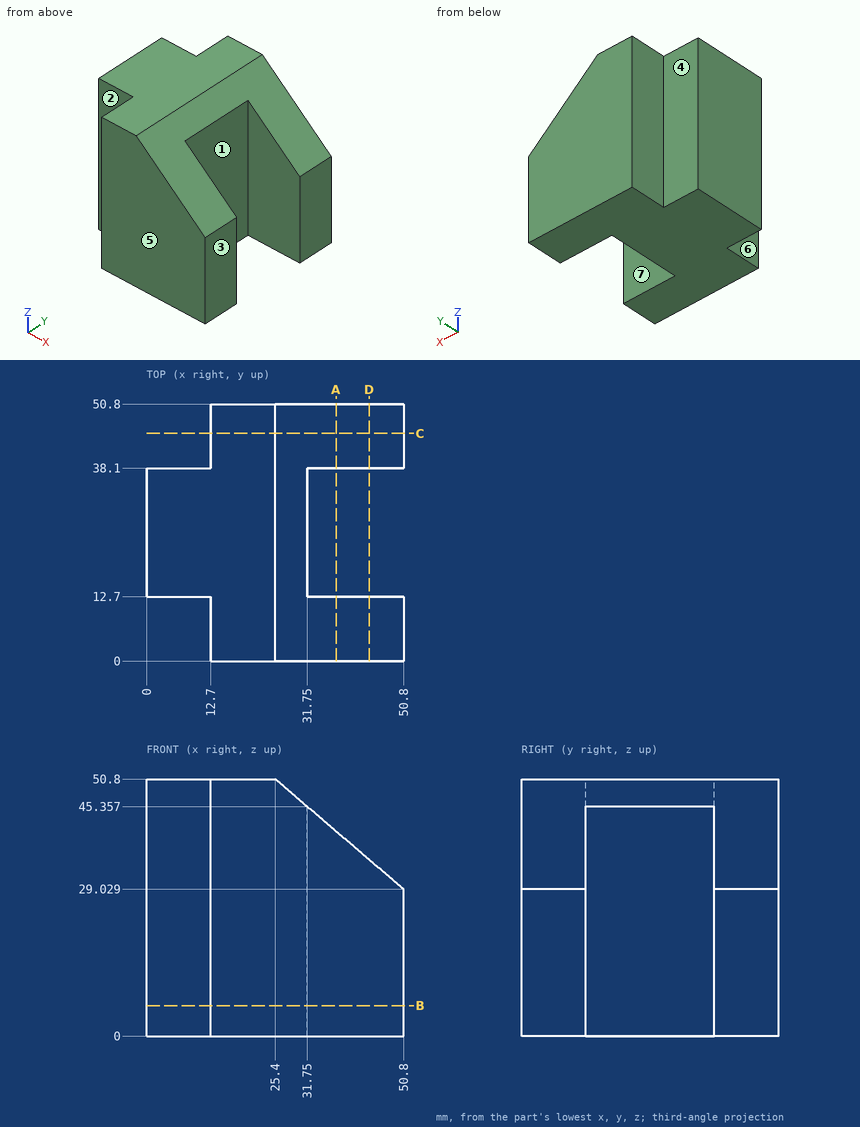
The drawing under review shows one solid part. Ordinate dimensions are in mm from its lowest x, y, z. A direction names the side the tool comes from. Coordinates: 2 decimals unless noted, no trailing zeros. Write each loop counter-clockwise with the first axis right and the second up, starting at its lowest first coordinate (ties: lowest second). Pieces come first, ordered by that corner, then holes. Notation, with made-up numbers: (57, 65) -> (102, 65) arc R28 cw to (102, 89) -> close; hole circle Ø4 at (38.5, -15). An arc over 180 degrees is marked (long way). One line per item, written item: value. Start each with the question number.
Q1. The part is to be moulded in two halves that separate along Y. For the marked faces 1, 2 and 3, say which applies: +Y half, -Y half, draft (parallel to the pull), parting line (faces both ways), or undercut.
Q2. Add section C-C, the plane y = 45. Give the boundary of the cut face in (x, z).
Q3. Clearance check with flat-ended pins moving along their axes: P1, Ø1.5, axis at x = 5.5, z = 25, coming from the +Y side; P2, Ø5, axis at y = 5, z = 27, coming from the -X side; P3, Ø20.5, axis at y = 23, z = 18, coming from the +X side. State where each tip first meets the part, or that it passes through.
Q4. To check wall thickness, follow probe 1 along Y at (x, z) = (44, 19.5); probe 2 along X at (y, z) = (13, 28); probe 3 along X at (y, z) = (7, 4). State the ranges of each line that lie inside material, in increasing order.
Q5. Add section D-D, the plane x = 44. Give the boundary of the cut face in (y, z).
Q6. Add section B-B, the plane z = 6. Give the boundary of the cut face in (x, y), then the cut area to 3 significant figures.
Q7. Add section A-A, the plane x = 37.5. Give the boundary of the cut face in (y, z), then the cut area to 3 significant figures.
Q8. For the marked faces 4, 5, 6 and 7, list the 3-axis set-ups (+Z, -Z, +X, -X, +Y, -Y) from which the entire face can be reached by the end or side of a thin tool; tool diameter is ignored.
Response:
1. face 1: undercut
1. face 2: -Y half
1. face 3: draft
2. outline: (12.7, 0) -> (50.8, 0) -> (50.8, 29.03) -> (25.4, 50.8) -> (12.7, 50.8) -> close
3. P1: y = 38.1
3. P2: x = 12.7
3. P3: x = 31.75
4. probe 1: 0 to 12.7, 38.1 to 50.8
4. probe 2: 0 to 31.75
4. probe 3: 12.7 to 50.8
5. outline: (0, 0) -> (12.7, 0) -> (12.7, 34.86) -> (0, 34.86) -> close; (38.1, 0) -> (50.8, 0) -> (50.8, 34.86) -> (38.1, 34.86) -> close
6. outline: (0, 12.7) -> (12.7, 12.7) -> (12.7, 0) -> (50.8, 0) -> (50.8, 12.7) -> (31.75, 12.7) -> (31.75, 38.1) -> (50.8, 38.1) -> (50.8, 50.8) -> (12.7, 50.8) -> (12.7, 38.1) -> (0, 38.1) -> close
6. area: 1,770 mm²
7. outline: (0, 0) -> (12.7, 0) -> (12.7, 40.43) -> (0, 40.43) -> close; (38.1, 0) -> (50.8, 0) -> (50.8, 40.43) -> (38.1, 40.43) -> close
7. area: 1,030 mm²
8. face 4: +Z, -Z, -X, +Y
8. face 5: +Z, -Z, +X, -X, -Y
8. face 6: +Z, -Z, -X, -Y
8. face 7: +Z, -Z, +X
